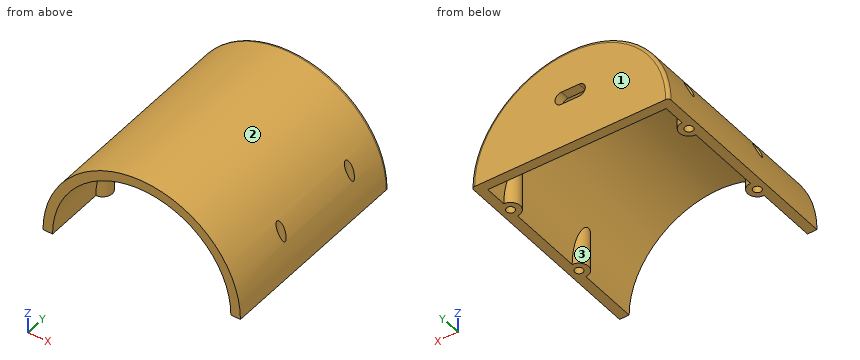
from build123d import *

# Parameters (mm, degrees)
EXTRUDE_1_DEPTH     = 65
EXTRUDE_5_REACH     = 80.403
SKETCH_12_R         = 3
SKETCH_16_R         = 1.3
CUT_EXTRUDE_2_DEPTH = 79.402806155
EXTRUDE_START       = -3
EXTRUDE_6_DEPTH     = 3
FILLET_1_R          = 1
CUT_EXTRUDE_3_REACH = 80.403


with BuildPart() as part:
    # Эскиз1 → Бобышка-Вытянуть1 (new body)
    with BuildSketch(Plane(origin=(0, 0, 0), x_dir=(1, 0, 0), z_dir=(0, 1, 0))):
        with BuildLine():
            Line((-31, 0), (-28, 0))
            ThreePointArc((-28, 0), (0, -28), (28, 0))
            Line((28, 0), (31, 0))
            ThreePointArc((31, 0), (0, -31), (-31, 0))
        make_face()
    extrude(amount=EXTRUDE_1_DEPTH)

    # Эскиз12 → Бобышка-Вытянуть5 (add, up to next)
    with BuildSketch(Plane(origin=(0, 0, 0), x_dir=(-1, 0, 0), z_dir=(0, 0, -1)), mode=Mode.PRIVATE) as extrude_5_sk1:
        with Locations((28, 52)):
            Circle(SKETCH_12_R)
    extrude_5_tool1 = extrude(extrude_5_sk1.sketch, amount=-EXTRUDE_5_REACH, mode=Mode.PRIVATE) - part.part
    # Эскиз12 → Бобышка-Вытянуть5 (add, up to next)
    with BuildSketch(Plane(origin=(0, 0, 0), x_dir=(-1, 0, 0), z_dir=(0, 0, -1)), mode=Mode.PRIVATE) as extrude_5_sk2:
        with Locations((28, 22)):
            Circle(SKETCH_12_R)
    extrude_5_tool2 = extrude(extrude_5_sk2.sketch, amount=-EXTRUDE_5_REACH, mode=Mode.PRIVATE) - part.part
    # Эскиз12 → Бобышка-Вытянуть5 (add, up to next)
    with BuildSketch(Plane(origin=(0, 0, 0), x_dir=(-1, 0, 0), z_dir=(0, 0, -1)), mode=Mode.PRIVATE) as extrude_5_sk3:
        with Locations((-28, 52)):
            Circle(SKETCH_12_R)
    extrude_5_tool3 = extrude(extrude_5_sk3.sketch, amount=-EXTRUDE_5_REACH, mode=Mode.PRIVATE) - part.part
    # Эскиз12 → Бобышка-Вытянуть5 (add, up to next)
    with BuildSketch(Plane(origin=(0, 0, 0), x_dir=(-1, 0, 0), z_dir=(0, 0, -1)), mode=Mode.PRIVATE) as extrude_5_sk4:
        with Locations((-28, 22)):
            Circle(SKETCH_12_R)
    extrude_5_tool4 = extrude(extrude_5_sk4.sketch, amount=-EXTRUDE_5_REACH, mode=Mode.PRIVATE) - part.part
    add(extrude_5_tool1.solids().sort_by_distance((-28, 52, 0))[0])
    add(extrude_5_tool2.solids().sort_by_distance((-28, 22, 0))[0])
    add(extrude_5_tool3.solids().sort_by_distance((28, 52, 0))[0])
    add(extrude_5_tool4.solids().sort_by_distance((28, 22, 0))[0])

    # Эскиз16 → Вырез-Вытянуть2 (cut, through all)
    with BuildSketch(Plane(origin=(0, 0, 0), x_dir=(-1, 0, 0), z_dir=(0, 0, -1))):
        with Locations((28, 52)):
            Circle(SKETCH_16_R)
        with Locations((28, 22)):
            Circle(SKETCH_16_R)
        with Locations((-28, 22)):
            Circle(SKETCH_16_R)
        with Locations((-28, 52)):
            Circle(SKETCH_16_R)
    extrude(amount=-CUT_EXTRUDE_2_DEPTH, mode=Mode.SUBTRACT)

    # Эскиз2 → Бобышка-Вытянуть6 (add)
    with BuildSketch(Plane(origin=(0, 65, 0), x_dir=(1, 0, 0), z_dir=(0, 1, 0)).offset(EXTRUDE_START)):
        with BuildLine():
            Line((-31, 0), (31, 0))
            ThreePointArc((31, 0), (0, -31), (-31, 0))
        make_face()
    extrude(amount=EXTRUDE_6_DEPTH)

    # Скругление1
    fillet_1_edges = [part.edges().sort_by_distance(p)[0] for p in [
        (0, 65, 31),
    ]]
    fillet(fillet_1_edges, radius=FILLET_1_R)

    # Эскиз18 → Вырез-Вытянуть3 (cut, up to next)
    with BuildSketch(Plane(origin=(0, 65, 0), x_dir=(1, 0, 0), z_dir=(0, 1, 0)), mode=Mode.PRIVATE) as cut_extrude_3_sk1:
        with BuildLine():
            Line((-2.75, -14.13), (2.75, -14.13))
            ThreePointArc((2.75, -14.13), (4.75, -16.13), (2.75, -18.13))
            Line((2.75, -18.13), (-2.75, -18.13))
            ThreePointArc((-2.75, -18.13), (-4.75, -16.13), (-2.75, -14.13))
        make_face()
    cut_extrude_3_tool1 = extrude(cut_extrude_3_sk1.sketch, amount=-CUT_EXTRUDE_3_REACH, mode=Mode.PRIVATE) & part.part
    add(cut_extrude_3_tool1.solids().sort_by_distance((0, 65, 16.13))[0], mode=Mode.SUBTRACT)


solid = part.part
Source: CAD feature listing. Evaluate the final solid. Frame: model axes, mm. Face numbers are marked on the shaded views. Coordinates: 2 decimals unless noted, no trailing zeros. Loops run counter-clockwise (first coordinate to the right, second up) from the corner with the lowest first, then second, coordinate; pieces in that order, holes last. Notation, with made-up numbers: M 5.25,-25.75 L 61.25,-25.75 A23 cw 61.25,-17.75 Z; hole C 28.25,-17.5 d2. An arc over 180 degrees is marked long. Answer in a Markdown table with one row per item.
Q1. Section A-A on y = 52. Return the cut outline in (x, z).
Answers below:
| item | result |
|---|---|
| outline | M -31,0 L -29.3,0 L -29.3,10.12 A31 ccw Z; M -26.7,0 L -25,0 L -25,12.61 A28 cw 25,12.61 L 25,0 L 26.7,0 L 26.7,15.75 A31 ccw -26.7,15.75 Z; M 29.3,0 L 31,0 A31 ccw 29.3,10.12 Z |
Q2. Section B-B on y = 40. Return the cut outline in (x, z), plus the area to 3 significant figures.
Answers below:
| item | result |
|---|---|
| outline | M -31,0 L -28,0 A28 cw 28,0 L 31,0 A31 ccw Z |
| area | 278 mm^2 |
Q3. Draft query along X for the marked faces 1, 2 and 3. Return one class per face: pulls with the +X half, pulls with the -X half, needs draft (parallel to the pull), parting line crosses it, or undercut.
Answers below:
| item | result |
|---|---|
| face 1 | needs draft |
| face 2 | parting line crosses it |
| face 3 | undercut |
Q4. First-contact query: pin 1 (8 mm diameter, centred on x = -8.5, y = 47.5, fed in from +Z); pin 2 (2 mm diameter, centred on x = -1, y = 46.5, fed in from -Z); pin 3 (4 mm diameter, centred on x = 28, y = 22, fed in from -Z); pin 4 (2.5 mm diameter, centred on x = 1.5, y = 63.5, fed in from +Z). Flat tips, straight axial feed; report the tip coordinate or a pass-through.
Answers below:
| item | result |
|---|---|
| pin 1 | stops at z = 30.67 |
| pin 2 | stops at z = 27.93 |
| pin 3 | stops at z = 0 |
| pin 4 | stops at z = 31 |
Q5. Ray query, probe 1 along Y at (x, z) = (-28, 5); probe 2 along X at (y, z) = (22, 11); probe 3 along X at (y, z) = (8, 1). Return the intervals inside material, ascending. Write a range as from..to.
Answers below:
| item | result |
|---|---|
| probe 1 | y = 0..20.7, 23.3..50.7, 53.3..65 |
| probe 2 | x = -26.7..-25, 25..26.7 |
| probe 3 | x = -30.98..-27.98, 27.98..30.98 |
Q6. Section C-C on z = 2. State how many separate pieces and enclosed holes the cut face has, plus the area to 3 significant figures.
Answers below:
| item | result |
|---|---|
| separate pieces | 1 |
| enclosed holes | 4 |
| area | 592 mm^2 |
